The model under review builds one solid part; all positions refer to its coordinate system, in mm. A direction names the side the tool comes from. Round coordinates to 2 decimals unless told otherwise and drop trailing zeros. Loops run counter-clockwise (first coordinate to the right, second up) from the corner with the lowest first, then second, coordinate; pieces in that order, holes last. Notation, with made-up numbers: M -19,21.5 L 13,21.5 A19 cw 13,36.5 Z; hole C 59.5,20 d11. An arc over 180 degrees is marked long. One line per question, with ' | ' between items.
from build123d import *

# Parameters (mm, degrees)
SKETCH_1_W          = 60
SKETCH_1_H          = 33
EXTRUDE_1_DEPTH     = 77
CUT_EXTRUDE_1_DEPTH = 73
SKETCH_3_R          = 1.7
CUT_EXTRUDE_2_DEPTH = 34
CUT_EXTRUDE_3_DEPTH = 61
SKETCH_5_W          = 10
SKETCH_5_H          = 15.5
CUT_EXTRUDE_4_DEPTH = 5
FILLET_1_R          = 1


with BuildPart() as part:
    # ｽｹｯﾁ1 → ﾎﾞｽ - 押し出し1 (new body)
    with BuildSketch(Plane(origin=(0, 0, 0), x_dir=(1, 0, 0), z_dir=(0, 1, 0))):
        Rectangle(SKETCH_1_W, SKETCH_1_H)
    extrude(amount=EXTRUDE_1_DEPTH)

    # ｽｹｯﾁ2 → ｶｯﾄ - 押し出し1 (cut)
    with BuildSketch(Plane.XZ):
        with BuildLine():
            Line((12.75, 13.75), (-12.75, 13.75))
            ThreePointArc((-12.75, 13.75), (-16.992640687, 11.992640687), (-18.75, 7.75))
            Line((-18.75, 7.75), (-18.75, -7.75))
            ThreePointArc((-18.75, -7.75), (-16.992640687, -11.992640687), (-12.75, -13.75))
            Line((-12.75, -13.75), (12.75, -13.75))
            ThreePointArc((12.75, -13.75), (16.992640687, -11.992640687), (18.75, -7.75))
            Line((18.75, -7.75), (18.75, 7.75))
            ThreePointArc((18.75, 7.75), (16.992640687, 11.992640687), (12.75, 13.75))
        make_face()
    extrude(amount=-CUT_EXTRUDE_1_DEPTH, mode=Mode.SUBTRACT)

    # ｽｹｯﾁ3 → ｶｯﾄ - 押し出し2 (cut, through all)
    with BuildSketch(Plane.XY.offset(16.5)):
        with Locations((26.25, 3.5)):
            Circle(SKETCH_3_R)
        with Locations((26.25, 67)):
            Circle(SKETCH_3_R)
        with Locations((-26.25, 67)):
            Circle(SKETCH_3_R)
        with Locations((-26.25, 3.5)):
            Circle(SKETCH_3_R)
    extrude(amount=-CUT_EXTRUDE_2_DEPTH, mode=Mode.SUBTRACT)

    # ｽｹｯﾁ4 → ｶｯﾄ - 押し出し3 (cut, through all)
    with BuildSketch(Plane.ZY.offset(30)):
        with BuildLine():
            Line((6.5, 40), (-6.5, 40))
            ThreePointArc((-6.5, 40), (-10.742640687, 38.242640687), (-12.5, 34))
            Line((-12.5, 34), (-12.5, 0))
            Line((-12.5, 0), (12.5, 0))
            Line((12.5, 0), (12.5, 34))
            ThreePointArc((12.5, 34), (10.742640687, 38.242640687), (6.5, 40))
        make_face()
    extrude(amount=-CUT_EXTRUDE_3_DEPTH, mode=Mode.SUBTRACT)

    # ｽｹｯﾁ5 → ｶｯﾄ - 押し出し4 (cut, through all)
    with BuildSketch(Plane.XZ.offset(-73)):
        with Locations((7.75, 0)):
            Rectangle(SKETCH_5_W, SKETCH_5_H)
    extrude(amount=-CUT_EXTRUDE_4_DEPTH, mode=Mode.SUBTRACT)

    # ﾌｨﾚｯﾄ1
    fillet_1_edges = [part.edges().sort_by_distance(p)[0] for p in [
        (30, 77, 0),
        (0, 77, -16.5),
        (-30, 77, 0),
        (0, 77, 16.5),
    ]]
    fillet(fillet_1_edges, radius=FILLET_1_R)


solid = part.part
1) Add section C-C on y = 30.5. State the section outline as (x, z) points, then the cut area to 3 significant figures.
Output values:
outline: M -30,-16.5 L 30,-16.5 L 30,-12.5 L 16.42,-12.5 A6 cw 12.75,-13.75 L -12.75,-13.75 A6 cw -16.42,-12.5 L -30,-12.5 Z; M -30,12.5 L -16.42,12.5 A6 cw -12.75,13.75 L 12.75,13.75 A6 cw 16.42,12.5 L 30,12.5 L 30,16.5 L -30,16.5 Z | area: 404 mm²
2) Add section A-A on y = 67. State the section outline as (x, z) points.
Output values:
outline: M -30,-16.5 L -27.95,-16.5 L -27.95,16.5 L -30,16.5 Z; M -24.55,-16.5 L 24.55,-16.5 L 24.55,16.5 L -24.55,16.5 Z; M 27.95,-16.5 L 30,-16.5 L 30,16.5 L 27.95,16.5 Z; hole M -18.75,-7.75 A6 ccw -12.75,-13.75 L 12.75,-13.75 A6 ccw 18.75,-7.75 L 18.75,7.75 A6 ccw 12.75,13.75 L -12.75,13.75 A6 ccw -18.75,7.75 Z
3) Add section B-B on x = -26.25. State the section outline as (y, z) points.
Output values:
outline: M 0,-16.5 L 1.8,-16.5 L 1.8,-12.5 L 0,-12.5 Z; M 0,12.5 L 1.8,12.5 L 1.8,16.5 L 0,16.5 Z; M 5.2,-16.5 L 65.3,-16.5 L 65.3,16.5 L 5.2,16.5 L 5.2,12.5 L 34,12.5 A6 cw 40,6.5 L 40,-6.5 A6 cw 34,-12.5 L 5.2,-12.5 Z; M 68.7,-16.5 L 76,-16.5 A1 ccw 77,-15.5 L 77,15.5 A1 ccw 76,16.5 L 68.7,16.5 Z
4) Machinability: for faces 4 (the cylindrical face through (23.113, 38.196, 10.789)), 5 (the flat face through (8, 75, -7.75)), 6 (the flat face through (0, 36, -13.75)), 7 (the flat face through (0, 37, 16.5)), which of the approach directions +Z, -Z, +X, -X, +Y, -Y give a long, thin tool a straight path to every point of the face, cutting with its end or side? Answer none if there is none.
Output values:
face 4: +X, -X, -Y | face 5: +Y, -Y | face 6: -Y | face 7: +Z, +X, -X, +Y, -Y
5) Insertion check: P1, Ø5.5, axis at x = 26.5, z = 1, coming from the -Y side; P2, Ø1.5, axis at x = 10.5, z = 10, coming from the -Y side. Each pin has a flat end and moves straight along its axis. Give the tip position at first contact, or say it passes through.
Output values:
P1: stops at y = 40 | P2: stops at y = 73
6) For line 1 (Y direction, x = 26.25, z = 13.6); line 2 (X direction, y = 67, z = 8); line 3 (X direction, y = 49, z = -8), list the stretches that pass through material, from the lowest coordinate up.
Output values:
line 1: y = 0 to 1.8, 5.2 to 65.3, 68.7 to 77 | line 2: x = -30 to -27.95, -24.55 to -18.74, 18.74 to 24.55, 27.95 to 30 | line 3: x = -30 to -18.74, 18.74 to 30
7) Mouldability with a two-part tool opening along Y and no side actions: class faces 1 (the cylindrical face through (-24.7, 2.8, -14.5)), 2 (the flat face through (0, 0, 15)), 3 (the flat face through (12.75, 75, 0)) as +Y half, -Y half, draft (parallel to the pull), parting line (faces both ways), or undercut.
Output values:
face 1: undercut | face 2: -Y half | face 3: draft
8) Add section D-D on y = 3.5. State how many separate pieces and enclosed holes the cut face has, then the cut area to 3 significant figures.
Output values:
separate pieces: 6 | enclosed holes: 0 | area: 349 mm²
